Build history of the part. All positions in model axes, mm. A direction names the side the tool comes from. Round coordinates to 2 decimals unless told otherwise and drop trailing zeros. Loops run counter-clockwise (first coordinate to the right, second up) from the corner with the lowest first, then second, coordinate; pieces in that order, holes last. Notation, with made-up numbers: M -7.75,5.25 L 1.25,5.25 A23 cw 1.25,26.25 Z; hole C -21.75,43.25 d8. An arc over 180 degrees is marked long. Use one line per item in the form item = value. Start each with the question number.
```python
from build123d import *

# Parameters (mm, degrees)
BOSS_EXTRUDE1_DEPTH     = 212
CUT_EXTRUDE1_REACH      = 92.491
SKETCH2_W               = 17.02
SKETCH2_H               = 10
SKETCH3_R               = 1.5
CUT_EXTRUDE2_DEPTH      = 15
SKETCH4_R               = 3
CUT_EXTRUDE3_DEPTH      = 111.491488024
CUT_EXTRUDE3_DEPTH_BACK = 1
SKETCH5_W               = 30
SKETCH5_H               = 15
CUT_EXTRUDE4_DEPTH      = 15
SKETCH6_R               = 3
CUT_EXTRUDE5_DEPTH      = 15.491488024
CUT_EXTRUDE5_DEPTH_BACK = 97
BOSS_EXTRUDE2_DEPTH     = 10
BOSS_EXTRUDE3_DEPTH     = 10
SKETCH9_W               = 40
SKETCH9_H               = 6.35
CUT_EXTRUDE6_DEPTH      = 1
CUT_EXTRUDE6_DEPTH_BACK = 213
CUT_EXTRUDE9_DEPTH      = 25
CUT_EXTRUDE9_DEPTH_BACK = 27
SKETCH11_R              = 7.5
CUT_EXTRUDE10_DEPTH     = 101.491488024
SKETCH12_R              = 4
CUT_EXTRUDE11_DEPTH     = 44.22
FILLET2_R               = 10
FILLET3_R               = 3


with BuildPart() as part:
    # Sketch1 → Boss-Extrude1 (new body)
    with BuildSketch(Plane.XY):
        Polygon((0, 0), (0, -6), (-17.02, -6), (-118.8, 8.518342212), (-118.8, -66), (-17.02, -66), (-17.02, -71), (0, -71), (0, -76), (-130.862615106, -76), (-147.02, -96), (-167.02, -96), (-167.02, -86), (-118.611740262, 14.491488024), (-17.02, 0), align=None)
    extrude(amount=BOSS_EXTRUDE1_DEPTH)

    # Sketch2 → Cut-Extrude1 (cut, up to next)
    with BuildSketch(Plane.XZ.offset(76), mode=Mode.PRIVATE) as cut_extrude1_sk1:
        with Locations((-8.51, 207)):
            Rectangle(SKETCH2_W, SKETCH2_H)
    cut_extrude1_tool1 = extrude(cut_extrude1_sk1.sketch, amount=-CUT_EXTRUDE1_REACH, mode=Mode.PRIVATE) & part.part
    add(cut_extrude1_tool1.solids().sort_by_distance((-8.51, -76, 207))[0], mode=Mode.SUBTRACT)
    # Sketch2 → Cut-Extrude1 (cut, up to next)
    with BuildSketch(Plane.XZ.offset(76), mode=Mode.PRIVATE) as cut_extrude1_sk2:
        with Locations((-8.51, 5)):
            Rectangle(SKETCH2_W, SKETCH2_H)
    cut_extrude1_tool2 = extrude(cut_extrude1_sk2.sketch, amount=-CUT_EXTRUDE1_REACH, mode=Mode.PRIVATE) & part.part
    add(cut_extrude1_tool2.solids().sort_by_distance((-8.51, -76, 5))[0], mode=Mode.SUBTRACT)

    # Sketch3 → Cut-Extrude2 (cut)
    with BuildSketch(Plane(origin=(-118.8, 0, 0), x_dir=(0, 0, -1), z_dir=(1, 0, 0))):
        with Locations((-159.5, -8.731657788)):
            Circle(SKETCH3_R)
        with Locations((-159.5, -48.731657788)):
            Circle(SKETCH3_R)
        with Locations((-52.5, -48.731657788)):
            Circle(SKETCH3_R)
        with Locations((-52.5, -8.731657788)):
            Circle(SKETCH3_R)
    extrude(amount=-CUT_EXTRUDE2_DEPTH, mode=Mode.SUBTRACT)

    # Sketch4 → Cut-Extrude3 (cut, two sides)
    with BuildSketch(Plane(origin=(0, -96, 0), x_dir=(1, 0, 0), z_dir=(0, 1, 0))) as cut_extrude3_sk:
        with Locations((-157.02, -187)):
            Circle(SKETCH4_R)
        with Locations((-157.02, -25)):
            Circle(SKETCH4_R)
    extrude(amount=CUT_EXTRUDE3_DEPTH, mode=Mode.SUBTRACT)
    extrude(cut_extrude3_sk.sketch, amount=-CUT_EXTRUDE3_DEPTH_BACK, mode=Mode.SUBTRACT)

    # Sketch5 → Cut-Extrude4 (cut)
    with BuildSketch(Plane(origin=(0, -66, 0), x_dir=(1, 0, 0), z_dir=(0, 1, 0))):
        with Locations((-98.8, -184.31184426)):
            Rectangle(SKETCH5_W, SKETCH5_H)
    extrude(amount=-CUT_EXTRUDE4_DEPTH, mode=Mode.SUBTRACT)

    # Sketch6 → Cut-Extrude5 (cut, two sides)
    with BuildSketch(Plane(origin=(0, 0, 0), x_dir=(1, 0, 0), z_dir=(0, 1, 0))) as cut_extrude5_sk:
        with Locations((-8.52, -30)):
            Circle(SKETCH6_R)
        with Locations((-8.52, -182)):
            Circle(SKETCH6_R)
    extrude(amount=CUT_EXTRUDE5_DEPTH, mode=Mode.SUBTRACT)
    extrude(cut_extrude5_sk.sketch, amount=-CUT_EXTRUDE5_DEPTH_BACK, mode=Mode.SUBTRACT)

    # Sketch7 → Boss-Extrude2 (add)
    with BuildSketch(Plane.XY.offset(212)):
        Polygon((-17.02, 0), (-118.611740262, 14.491488024), (-167.02, -86), (-167.02, -96), (-17.02, -96), align=None)
    extrude(amount=-BOSS_EXTRUDE2_DEPTH)

    # Sketch8 → Boss-Extrude3 (add)
    with BuildSketch(Plane(origin=(0, 0, 0), x_dir=(-1, 0, 0), z_dir=(0, 0, -1))):
        Polygon((167.02, -86), (167.02, -96), (17.02, -96), (17.02, 0), (118.611740262, 14.491488024), align=None)
    extrude(amount=-BOSS_EXTRUDE3_DEPTH)

    # Sketch9 → Cut-Extrude6 (cut, two sides)
    with BuildSketch(Plane.XY.offset(212)) as cut_extrude6_sk:
        with Locations((-59.52, -92.825)):
            Rectangle(SKETCH9_W, SKETCH9_H)
    extrude(amount=CUT_EXTRUDE6_DEPTH, mode=Mode.SUBTRACT)
    extrude(cut_extrude6_sk.sketch, amount=-CUT_EXTRUDE6_DEPTH_BACK, mode=Mode.SUBTRACT)

    # Sketch10 → Cut-Extrude9 (cut, two sides)
    with BuildSketch(Plane(origin=(0, 0, 0), x_dir=(1, 0, 0), z_dir=(0, 1, 0))) as cut_extrude9_sk:
        with BuildLine():
            Line((-17.02, -140.641016151), (-17.02, -71.358983849))
            ThreePointArc((-17.02, -71.358983849), (-77.02, -106), (-17.02, -140.641016151))
        make_face()
    extrude(amount=CUT_EXTRUDE9_DEPTH, mode=Mode.SUBTRACT)
    extrude(cut_extrude9_sk.sketch, amount=-CUT_EXTRUDE9_DEPTH_BACK, mode=Mode.SUBTRACT)

    # Sketch11 → Cut-Extrude10 (cut, through all)
    with BuildSketch(Plane(origin=(0, -86, 0), x_dir=(-1, 0, 0), z_dir=(0, -1, 0))):
        with Locations((157.02, -25)):
            Circle(SKETCH11_R)
        with Locations((157.02, -187)):
            Circle(SKETCH11_R)
    extrude(amount=-CUT_EXTRUDE10_DEPTH, mode=Mode.SUBTRACT)

    # Sketch12 → Cut-Extrude11 (cut, through all)
    with BuildSketch(Plane(origin=(-123.8, 0, 0), x_dir=(0, 0, -1), z_dir=(1, 0, 0))):
        with Locations((-159.5, -8.731657788)):
            Circle(SKETCH12_R)
        with Locations((-52.5, -8.731657788)):
            Circle(SKETCH12_R)
    extrude(amount=-CUT_EXTRUDE11_DEPTH, mode=Mode.SUBTRACT)

    # Fillet2
    fillet2_edges = [part.edges().sort_by_distance(p)[0] for p in [
        (-118.611740262, 14.491488024, 106),
    ]]
    fillet(fillet2_edges, radius=FILLET2_R)

    # Fillet3
    fillet3_edges = [part.edges().sort_by_distance(p)[0] for p in [
        (0, 0, 106),
    ]]
    fillet(fillet3_edges, radius=FILLET3_R)


solid = part.part
```
Q1. Drop flat-ended pins along their axis: P1, Ø9.5, axis at x = -157.02, z = 25, coming from the +Y side; P2, Ø5, axis at x = -95, z = 170, coming from the -Y side; P3, Ø5, axis at y = -91.5, z = 4.5, coming from the +X side; P4, Ø24, axis at x = -157.02, z = 25, coming from the -Y side. Give the stop position or say it passes through.
Q2. Saw through at C-C (z = 105.5). Give the cut face in (x, y), and give its area (3 significant figures).
Q3. Tool access for faces 1 (the face through (-77, 2.9, 104.8)), 2 (the face through (-60, -89.65, 5)), 3 (the face through (-9, -71, 105)), 4 (the face through (-9, -74, 202)): list every direction of +Z, -Z, +X, -X, +Y, -Y with a clear straight run to the whole face (end or side of a thin tool).
Q4. Wall check: probe 1 along Z at (x, y) = (-25, -5.5); probe 2 along Z at (x, y) = (-8.52, -73.95); probe 3 along Y at (x, z) = (-126.5, 159.5). Give the ranges that are in metal, low to high.
Q5. Saw through at B-B (z = 149). Give the cut face in (x, y), and give its area (3 significant figures).
Q6. Pull direction X, two halves, no side cores. Call faces 5 (the face through (-39.52, -93, 207)), 6 (the face through (-10, 0, 105)), 7 (the face through (-123.8, -10.5, 52.6)), 8 (the face through (-8.911, -2.958, 179.026)): pulls with the +X half, pulls with the -X half, needs draft (parallel to the pull), parting line crosses it, or undercut.
Q7. Saw through at D-D (y = -57). Give the cut face in (x, z).
Q8. Saw through at A-A (x = -8.52). Give the cut face in (y, z), and give its area (3 significant figures).
Filled in:
q1.P1 = -86
q1.P2 = -76
q1.P3 = -17.02
q1.P4 = -96
q2.outline = M -167.02,-96 L -147.02,-96 L -130.86,-76 L 0,-76 L 0,-71 L -17.02,-71 L -17.02,-66 L -118.8,-66 L -118.8,8.52 L -77.02,2.56 L -77.02,8.56 L -111.37,13.46 A10 ccw -121.79,7.9 L -167.02,-86 Z; M -17.02,-6 L 0,-6 L 0,-3 A3 ccw -3,0 L -17.02,0 Z
q2.area = 3,940 mm²
q3.face_1 = +Y
q3.face_2 = +Z, -Z, -Y
q3.face_3 = +Z, -Z, +X
q3.face_4 = +Z, +X, -Y
q4.probe_1 = 0 to 10, 202 to 212
q4.probe_2 = 10 to 27, 33 to 179, 185 to 202
q4.probe_3 = -76 to -50.23, -47.23 to -12.73, -4.73 to -1.88
q5.outline = M -167.02,-96 L -147.02,-96 L -130.86,-76 L 0,-76 L 0,-71 L -17.02,-71 L -17.02,-66 L -118.8,-66 L -118.8,8.52 L -17.02,-6 L 0,-6 L 0,-3 A3 ccw -3,0 L -17.02,0 L -111.37,13.46 A10 ccw -121.79,7.9 L -167.02,-86 Z
q5.area = 4,300 mm²
q6.face_5 = undercut
q6.face_6 = needs draft
q6.face_7 = pulls with the -X half
q6.face_8 = undercut
q7.outline = M -153.05,0 L -17.02,0 L -17.02,10 L -118.8,10 L -118.8,202 L -17.02,202 L -17.02,212 L -153.05,212 L -153.05,193.36 A7.5 cw -153.05,180.64 L -153.05,31.36 A7.5 cw -153.05,18.64 Z
q8.outline = M -76,10 L -71,10 L -71,27 L -76,27 Z; M -76,33 L -71,33 L -71,179 L -76,179 Z; M -76,185 L -71,185 L -71,202 L -76,202 Z; M -6,0 L 0,0 L 0,27 L -6,27 Z; M -6,33 L 0,33 L 0,179 L -6,179 Z; M -6,185 L 0,185 L 0,212 L -6,212 Z
q8.area = 2,100 mm²
